```python
from build123d import *

# Parameters (mm, degrees)
TOP_W                                     = 12
TOP_H                                     = 10
PRECISION_MICRODRIVES_MODEL_212_109_DEPTH = 24
TOP_RING_2_R                              = 2
TOP_RING_DEPTH                            = 0.7
HOLE_WIZARD_M1_1_D                        = 1.1
HOLE_WIZARD_M1_1_DEPTH                    = 10
HOLE_WIZARD_M1_1_TIP                      = 0.337040433
HOLE_WIZARD_M1_2_D                        = 1.1
HOLE_WIZARD_M1_2_DEPTH                    = 10
HOLE_WIZARD_M1_2_TIP                      = 0.337040433
D_SHAFT_DEPTH                             = 8
VERRUNDUNG1_R                             = 0.5
SKIZZE12_R                                = 2.5
BOTTOM_DEPTH                              = 1.2
SKIZZE13_R                                = 0.5
BOLT_DEPTH                                = 6
SKIZZE14_W                                = 0.12
SKIZZE14_H                                = 1.5
FLAPS_DEPTH                               = 2.5
FLAP1_CUT_REACH                           = 11.56
SKIZZE15_R                                = 0.4
FLAP2_CUT_REACH                           = 11.56
SKIZZE16_R                                = 0.4


with BuildPart() as part:
    # top → Precision Microdrives Model 212-109 (new body)
    with BuildSketch(Plane.XY):
        Rectangle(TOP_W, TOP_H)
    extrude(amount=-PRECISION_MICRODRIVES_MODEL_212_109_DEPTH)

    # top ring 2 → top-ring (add)
    with BuildSketch(Plane.XY):
        Circle(TOP_RING_2_R)
    extrude(amount=TOP_RING_DEPTH)

    # Hole Wizard M1-1
    with Locations(Plane.XY):
        with Locations((-4.5, 0)):
            Hole(HOLE_WIZARD_M1_1_D / 2, depth=HOLE_WIZARD_M1_1_DEPTH)
            with Locations((0, 0, -(HOLE_WIZARD_M1_1_DEPTH + HOLE_WIZARD_M1_1_TIP / 2))):  # 117° drill point
                Cone(0, HOLE_WIZARD_M1_1_D / 2, HOLE_WIZARD_M1_1_TIP, mode=Mode.SUBTRACT)

    # Hole Wizard M1-2
    with Locations(Plane.XY):
        with Locations((4.5, 0)):
            Hole(HOLE_WIZARD_M1_2_D / 2, depth=HOLE_WIZARD_M1_2_DEPTH)
            with Locations((0, 0, -(HOLE_WIZARD_M1_2_DEPTH + HOLE_WIZARD_M1_2_TIP / 2))):  # 117° drill point
                Cone(0, HOLE_WIZARD_M1_2_D / 2, HOLE_WIZARD_M1_2_TIP, mode=Mode.SUBTRACT)

    # Skizze11 → D-Shaft (add)
    with BuildSketch(Plane.XY):
        with BuildLine():
            Line((-1.071214264, 1.05), (1.071214264, 1.05))
            ThreePointArc((1.071214264, 1.05), (0, -1.5), (-1.071214264, 1.05))
        make_face()
    extrude(amount=D_SHAFT_DEPTH)

    # Verrundung1
    verrundung1_edges = [part.edges().sort_by_distance(p)[0] for p in [
        (-6, 5, -12),
        (6, 5, -12),
        (6, -5, -12),
        (-6, -5, -12),
    ]]
    fillet(verrundung1_edges, radius=VERRUNDUNG1_R)

    # Skizze12 → bottom (add)
    with BuildSketch(Plane(origin=(0, 0, -24), x_dir=(-1, 0, 0), z_dir=(0, 0, -1))):
        Circle(SKIZZE12_R)
    extrude(amount=BOTTOM_DEPTH)

    # Skizze13 → bolt (add)
    with BuildSketch(Plane(origin=(0, 0, -24), x_dir=(-1, 0, 0), z_dir=(0, 0, -1))):
        Circle(SKIZZE13_R)
    extrude(amount=BOLT_DEPTH)

    # Skizze14 → flaps (add)
    with BuildSketch(Plane(origin=(0, 0, -24), x_dir=(-1, 0, 0), z_dir=(0, 0, -1))):
        with Locations((-3.5, 0)):
            Rectangle(SKIZZE14_W, SKIZZE14_H)
        with Locations((3.5, 0)):
            Rectangle(SKIZZE14_W, SKIZZE14_H)
    extrude(amount=FLAPS_DEPTH)

    # Skizze15 → flap1-cut (cut, up to next)
    with BuildSketch(Plane.ZY.offset(3.56), mode=Mode.PRIVATE) as flap1_cut_sk1:
        with Locations((-25.7, 0)):
            Circle(SKIZZE15_R)
    flap1_cut_tool1 = extrude(flap1_cut_sk1.sketch, amount=-FLAP1_CUT_REACH, mode=Mode.PRIVATE) & part.part
    add(flap1_cut_tool1.solids().sort_by_distance((-3.56, 0, -25.7))[0], mode=Mode.SUBTRACT)

    # Skizze16 → flap2-cut (cut, up to next)
    with BuildSketch(Plane(origin=(3.56, 0, 0), x_dir=(0, 0, -1), z_dir=(1, 0, 0)), mode=Mode.PRIVATE) as flap2_cut_sk1:
        with Locations((25.7, 0)):
            Circle(SKIZZE16_R)
    flap2_cut_tool1 = extrude(flap2_cut_sk1.sketch, amount=-FLAP2_CUT_REACH, mode=Mode.PRIVATE) & part.part
    add(flap2_cut_tool1.solids().sort_by_distance((3.56, 0, -25.7))[0], mode=Mode.SUBTRACT)


solid = part.part
```
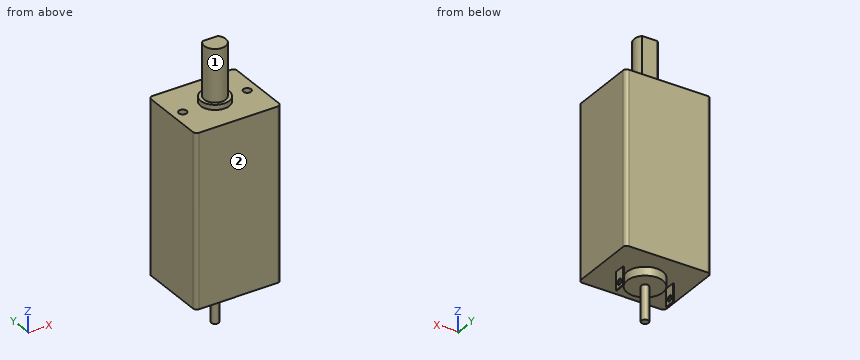
The listing builds one solid part. Answer for the finished solid, in the listing's coordinates (mm). Face numbers are marked on the shaded views. A direction names the side the tool comes from. Coordinates: 2 decimals unless noted, no trailing zeros. Write each loop counter-clockwise with the first axis right and the second up, starting at its lowest first coordinate (ties: lowest second). Pieces come first, ordered by that corner, then holes.
Q1. Section C-C, the plane x = 0 is taken. Write down the section's boundary in (y, z), then the cut area to 3 significant figures.
Returned:
outline: (-5, -24) - (-2.5, -24) - (-2.5, -25.2) - (-0.5, -25.2) - (-0.5, -30) - (0.5, -30) - (0.5, -25.2) - (2.5, -25.2) - (2.5, -24) - (5, -24) - (5, 0) - (2, 0) - (2, 0.7) - (1.05, 0.7) - (1.05, 8) - (-1.5, 8) - (-1.5, 0.7) - (-2, 0.7) - (-2, 0) - (-5, 0) - close
area: 272 mm2
Q2. Find the intervals of material crossed by line 1 along X through (y, z) = (0, -6); line 2 along Y through (x, z) = (-4.5, -6.5); line 3 along Y through (x, z) = (-3.5, -25.7), in increasing order.
Returned:
line 1: x = -6 to -5.05, -3.95 to 3.95, 5.05 to 6
line 2: y = -5 to -0.55, 0.55 to 5
line 3: y = -0.75 to -0.4, 0.4 to 0.75
Q3. Given P1, Ø0.8, axis at y = 0, z = -25.5, coming from the +X side; P2, Ø3, axis at x = -1.5, y = -1, coming from the -Z side; P3, Ø1.3, axis at x = 4.5, y = 0, coming from the -Z side; P4, Ø4, axis at x = -1, y = -2.5, coming from the -Z side, each flat-ended and moving along its own axis, determine where each tip first touches the part or whether it passes through.
Returned:
P1: stops at x = 3.56
P2: stops at z = -30
P3: stops at z = -24
P4: stops at z = -25.2
Q4. Section A-A, the plane z = -25.7 is taken. Write down the section's boundary in (x, y), then the cut area to 3 significant figures.
Returned:
outline: (-3.56, -0.75) - (-3.44, -0.75) - (-3.44, -0.4) - (-3.56, -0.4) - close; (-3.56, 0.4) - (-3.44, 0.4) - (-3.44, 0.75) - (-3.56, 0.75) - close; circle Ø1 at (0, 0); (3.44, -0.75) - (3.56, -0.75) - (3.56, -0.4) - (3.44, -0.4) - close; (3.44, 0.4) - (3.56, 0.4) - (3.56, 0.75) - (3.44, 0.75) - close
area: 0.953 mm2
Q5. Section B-B, the plane z = -0.5 is taken. Write down the section's boundary in (x, y).
Returned:
outline: (-6, -4.5) arc R0.5 ccw to (-5.5, -5) - (5.5, -5) arc R0.5 ccw to (6, -4.5) - (6, 4.5) arc R0.5 ccw to (5.5, 5) - (-5.5, 5) arc R0.5 ccw to (-6, 4.5) - close; hole circle Ø1.1 at (-4.5, 0); hole circle Ø1.1 at (4.5, 0)
Q6. Section D-D, the plane y = 3.5 is taken. Write down the section's boundary in (x, z), then the cut area to 3 significant figures.
Returned:
outline: (-6, -24) - (6, -24) - (6, 0) - (-6, 0) - close
area: 288 mm2
Q7. Which of the six approach directions +Z, -Z, +X, -X, +Y, -Y give full straight-line access (tool end or side, diameter ignored) to the marked faces 1 and 2?
Returned:
face 1: +Z
face 2: +Z, -Z, +X, -X, -Y
